Build history of the part. All positions in model axes, mm. A direction names the side the tool comes from. Round coordinates to 2 decimals unless told otherwise and drop trailing zeros. Order: outer loops, then holes, each group sorted by start corner. A loop starts at its lowest first (then second) coordinate and runs counter-clockwise, first axis right, second up. Notation, with made-up numbers: (-8.5, 75) - (42.5, 75) arc R21 ccw to (42.5, 100) - close; hole circle Ø4 at (82.25, 37). An arc over 180 degrees is marked (long way). Write each question's results on one line, items separated by ' | '. Start each with the question number.
```python
from build123d import *

# Parameters (mm, degrees)
SKETCH1_W           = 50.8
SKETCH1_H           = 25.4
SKETCH1_W_2         = 47.625
SKETCH1_H_2         = 23.8125
BOSS_EXTRUDE1_DEPTH = 457.2
SKETCH2_R           = 3.683
SKETCH2_W           = 26.416
SKETCH2_H           = 26.416
CUT_EXTRUDE1_DEPTH  = 26.4


with BuildPart() as part:
    # Sketch1 → Boss-Extrude1 (new body)
    with BuildSketch(Plane.XY):
        Rectangle(SKETCH1_W, SKETCH1_H)
        Rectangle(SKETCH1_W_2, SKETCH1_H_2, mode=Mode.SUBTRACT)
    extrude(amount=BOSS_EXTRUDE1_DEPTH)

    # Sketch2 → Cut-Extrude1 (cut, through all)
    with BuildSketch(Plane(origin=(0, 12.7, 0), x_dir=(1, 0, 0), z_dir=(0, 1, 0))):
        with Locations((0, -177.8)):
            Circle(SKETCH2_R)
        with Locations((0, -279.4)):
            Circle(SKETCH2_R)
        with Locations((0, -228.6)):
            Rectangle(SKETCH2_W, SKETCH2_H)
    extrude(amount=-CUT_EXTRUDE1_DEPTH, mode=Mode.SUBTRACT)


solid = part.part
```
1. Wall check: line 1 (Z direction, x = 0, y = -12.3); line 2 (Y direction, x = 16, z = 321.5); line 3 (X direction, y = -12.5, z = 177.8). Give the ranges that are in metal, low to high. Write a range as from..to.
2. Mould opens along Y. For faces 3 (the face through (-0.48, -12.3, 174.15)), 4 (the face through (16, 11.906, 225)), 5 (the face through (17, 12.7, 225)) say: pulls with the +Y half, pulls with the -Y half, needs draft (parallel to the pull), parting line crosses it, or undercut.
3. Cut at A-A (x = -17.5). List the corners of the cut face in (y, z).
4. Cut at B-B (y = -4.75). List the corners of the cut face in (x, z).
5. 3-axis set-ups, long thin cutter, end or side, ignore diameter. For faces 1 (the face through (-23.812, 0, 225)), 2 (the face through (-2, -12.2, 457.2)): which of +Z, -Z, +X, -X, +Y, -Y reach the whole face in a straight line?
6. Cut at C-C (z = 203). List the corners of the cut face in (x, y).
A:
1) line 1: z = 0..174.12, 181.48..215.39, 241.81..275.72, 283.08..457.2 | line 2: y = -12.7..-11.91, 11.91..12.7 | line 3: x = -25.4..-3.68, 3.68..25.4
2) face 3: needs draft | face 4: undercut | face 5: pulls with the +Y half
3) outline: (-12.7, 0) - (-11.91, 0) - (-11.91, 457.2) - (-12.7, 457.2) - close; (11.91, 0) - (12.7, 0) - (12.7, 457.2) - (11.91, 457.2) - close
4) outline: (-25.4, 0) - (-23.81, 0) - (-23.81, 457.2) - (-25.4, 457.2) - close; (23.81, 0) - (25.4, 0) - (25.4, 457.2) - (23.81, 457.2) - close
5) face 1: +Z, -Z | face 2: +Z, +X, -X, +Y, -Y
6) outline: (-25.4, -12.7) - (25.4, -12.7) - (25.4, 12.7) - (-25.4, 12.7) - close; hole (-23.81, -11.91) - (23.81, -11.91) - (23.81, 11.91) - (-23.81, 11.91) - close
